Read the model definition and answer for the solid it produces. Units are mm, in the model's axes. Face numbers are marked on the shaded views. A direction names the side the tool comes from. Coordinates: 2 decimals unless noted, no trailing zeros. Write each loop counter-clockwise with the first axis right and the second up, starting at its lowest first coordinate (ties: lowest second). Pieces come first, ordered by that corner, then holes. Notation, with made-up numbers: M 58,-17.75 L 111,-17.75 A29 cw 111,3.25 Z; hole C 63.25,77 d11. An arc over 180 degrees is marked long. Write item = value, one per line.
from build123d import *

# Parameters (mm, degrees)
F1_DEPTH = 25.4
F3_DEPTH = 19.05


with BuildPart() as f1:
    # F0 (on Front) → F1 (new body)
    with BuildSketch(Plane.XZ):
        Polygon((-25.4, 43.994091), (-47.397045, 31.294091), (-14.664697, -25.4), (50.8, -25.4), (50.8, 0), (0, 0), align=None)
    extrude(amount=F1_DEPTH)

    # F2 (on face) → F3 (cut)
    with BuildSketch(Plane.XZ.offset(25.4)):
        Polygon((-31.648493, 40.386522), (-42.647015, 34.036522), (-11.49801, -19.915138), (50.8, -19.915138), (50.8, -7.215138), (-4.165662, -7.215138), align=None)
    extrude(amount=-F3_DEPTH, mode=Mode.SUBTRACT)


solid = f1.part
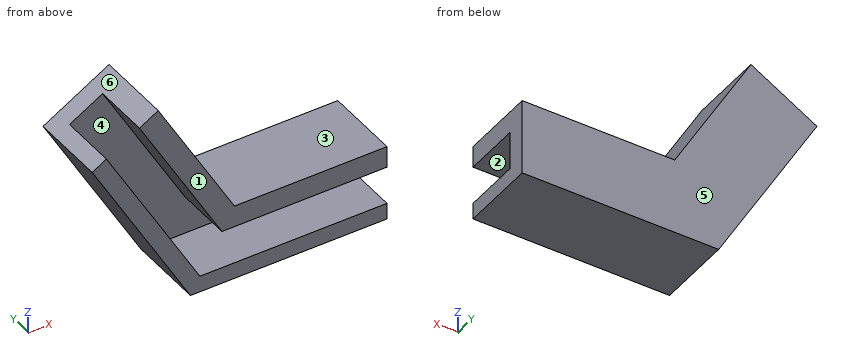
Item 1: Flat-ended cylindrical pins translate along their axes: pin 1 (12 mm diameter, centred on x = 20, y = -19.5, fed in from +Z); pin 2 (5 mm diameter, centred on y = -15.5, z = -1.5, fed in from -X); pin 3 (1 mm diameter, centred on x = -7.5, y = -17.5, fed in from +Z). Find the tip coordinate at first contact, or state that the pin passes through.
Worked answers:
pin_1 = 0
pin_2 = -29.91
pin_3 = 13.86
Item 2: Consider line 1 along Z through (x, y) = (28, -12.5); line 2 along Y through (x, z) = (-29, 35); line 3 along Z through (x, y) = (-20, -8). Determine where each line is inside the solid, lowest interval first. Write a range as from..to.
Worked answers:
line_1 = -25.4..-19.92, -7.22..0
line_2 = -6.35..0
line_3 = -16.16..-5.19, 20.21..34.64
Item 3: Find section A-A (y = -9.5). Determine the outline of the cut face in (x, z), and give its area (3 significant figures).
Worked answers:
outline = M -47.4,31.29 L -14.66,-25.4 L 50.8,-25.4 L 50.8,-19.92 L -11.5,-19.92 L -42.65,34.04 Z; M -31.65,40.39 L -4.17,-7.22 L 50.8,-7.22 L 50.8,0 L 0,0 L -25.4,43.99 Z
area = 1,460 mm²
Item 4: Find section C-C (z = -4.5). Determine the outline of the cut face in (x, y), and give its area (3 significant figures).
Worked answers:
outline = M -26.73,-25.4 L -20.4,-25.4 L -20.4,-6.35 L -5.73,-6.35 L -5.73,-25.4 L 50.8,-25.4 L 50.8,0 L -26.73,0 Z
area = 1,690 mm²
Item 5: Which of the six approach directions +Z, -Z, +X, -X, +Y, -Y give full straight-line access (tool end or side, diameter ignored) to the marked faces 1, 2 and 3?
Worked answers:
face_1 = +Z, -Z, +X, -X, -Y
face_2 = +X, -Y
face_3 = +Z, +X, +Y, -Y
Item 6: For a pull along Z with two mould halves and no side action, classify the marked faces 4, 5 and 6 as released by +Z, released by -Z, zero draft, split by the parting line, or undercut.
Worked answers:
face_4 = undercut
face_5 = zero draft
face_6 = released by +Z
Item 7: Find section B-B (x = 33.5). Determine the outline of the cut face in (y, z).
Worked answers:
outline = M -25.4,-25.4 L 0,-25.4 L 0,0 L -25.4,0 L -25.4,-7.22 L -6.35,-7.22 L -6.35,-19.92 L -25.4,-19.92 Z
